from build123d import *

# Parameters (mm, degrees)
SKETCH1_W             = 6.35
SKETCH1_H             = 25.4
BOSS_EXTRUDE1_DEPTH   = 6.604
BOSS_EXTRUDE1_2_DEPTH = 6.604
SKETCH2_W             = 38.608
SKETCH2_H             = 25.4
BOSS_EXTRUDE2_DEPTH   = 5.08
SKETCH3_W             = 13.97
SKETCH3_H             = 6.35
BOSS_EXTRUDE3_DEPTH   = 6.604
SKETCH4_R             = 2.159
CUT_EXTRUDE1_DEPTH    = 2.54
SKETCH5_R             = 1.7018
BOSS_EXTRUDE4_DEPTH   = 11.684
FILLET1_R             = 6.35
FILLET2_R             = 3.81
FILLET3_R             = 1.27


with BuildPart() as part:
    # Sketch1 → Boss-Extrude1 (new body)
    with BuildSketch(Plane(origin=(0, 0, 0), x_dir=(1, 0, 0), z_dir=(0, 1, 0))):
        with Locations((16.129, 12.7)):
            Rectangle(SKETCH1_W, SKETCH1_H)
    extrude(amount=BOSS_EXTRUDE1_DEPTH)



with BuildPart() as body_2:
    # Sketch1 → Boss-Extrude1 2 (new body)
    with BuildSketch(Plane(origin=(0, 0, 0), x_dir=(1, 0, 0), z_dir=(0, 1, 0))):
        with Locations((-16.129, 12.7)):
            Rectangle(SKETCH1_W, SKETCH1_H)
    extrude(amount=BOSS_EXTRUDE1_2_DEPTH)


with BuildPart() as part_1:
    add(part.part)

    add(body_2.part)  # Boss-Extrude2 merges body 2
    # Sketch2 → Boss-Extrude2 (add)
    with BuildSketch(Plane(origin=(0, 6.604, 0), x_dir=(1, 0, 0), z_dir=(0, 1, 0))):
        with Locations((0, 12.7)):
            Rectangle(SKETCH2_W, SKETCH2_H)
    extrude(amount=BOSS_EXTRUDE2_DEPTH)

    # Sketch3 → Boss-Extrude3 (add)
    with BuildSketch(Plane.XZ.offset(-6.604)):
        with Locations((0, -22.225)):
            Rectangle(SKETCH3_W, SKETCH3_H)
    extrude(amount=BOSS_EXTRUDE3_DEPTH)

    # Sketch4 → Cut-Extrude1 (cut)
    with BuildSketch(Plane.XY.offset(-19.05)):
        with Locations((3.81, 3.302)):
            Circle(SKETCH4_R)
        with Locations((-3.81, 3.302)):
            Circle(SKETCH4_R)
    extrude(amount=-CUT_EXTRUDE1_DEPTH, mode=Mode.SUBTRACT)

    # Sketch5 → Boss-Extrude4 (add)
    # profile 1 of 2: a face of its own
    with BuildSketch(Plane(origin=(0, 11.684, 0), x_dir=(1, 0, 0), z_dir=(0, 1, 0))):
        with BuildLine():
            Line((-19.304, 17.985297981), (-19.304, 7.414702019))
            ThreePointArc((-19.304, 7.414702019), (-30.335321913, 12.7), (-19.304, 17.985297981))
        make_face()
        with Locations(Location((-23.553521913, 12.7, 0), (0, 0, 270))):
            Circle(SKETCH5_R, mode=Mode.SUBTRACT)
    # profile 2 of 2: a face of its own
    with BuildSketch(Plane(origin=(0, 11.684, 0), x_dir=(1, 0, 0), z_dir=(0, 1, 0))):
        with BuildLine():
            Line((19.304, 17.985297981), (19.304, 7.414702019))
            ThreePointArc((19.304, 7.414702019), (30.335321913, 12.7), (19.304, 17.985297981))
        make_face()
        with Locations(Location((23.553521913, 12.7, 0), (0, 0, 270))):
            Circle(SKETCH5_R, mode=Mode.SUBTRACT)
    extrude(amount=-BOSS_EXTRUDE4_DEPTH)

    # Fillet1
    # the kernel refuses this fillet: 6.35 mm, written as the material it adds along each edge
    with BuildSketch(Plane(origin=(-19.304, 11.684, -7.414702019), x_dir=(0, 0, 1), z_dir=(0, -1, 0)), Plane(origin=(19.304, 11.684, -17.985297981), x_dir=(0, 0, -1), z_dir=(0, -1, 0))) as fillet1_piece_1:
        with BuildLine():
            CenterArc((7.678309884, 6.344526057), FILLET1_R, 189.180006139, 78.44078763)
            Line((1.409640703, 5.331467961), (1.28426732, 5.311206799))
            ThreePointArc((1.28426732, 5.311206799), (1.148418354, 2.548446621), (-0.098975618, 0.079579062))
            Line((-0.098975618, 0.079579062), (0, -0.127))
            ThreePointArc((0, -0.127), (3.707351009, -0.127), (7.409429861, -0.126890521))
            Line((7.409429861, -0.126890521), (7.414702019, 0))
        make_face()
    extrude(amount=11.684)
    with BuildSketch(Plane(origin=(-19.304, 11.684, -17.985297981), x_dir=(0, 0, -1), z_dir=(0, -1, 0)), Plane(origin=(19.304, 11.684, -7.414702019), x_dir=(0, 0, 1), z_dir=(0, -1, 0))) as fillet1_piece_2:
        with BuildLine():
            CenterArc((7.678309884, -6.344526057), FILLET1_R, 92.379206231, 78.44078763)
            Line((1.409640703, -5.331467961), (1.28426732, -5.311206799))
            ThreePointArc((1.28426732, -5.311206799), (1.148418354, -2.548446621), (-0.098975618, -0.079579062))
            Line((-0.098975618, -0.079579062), (0, 0.127))
            ThreePointArc((0, 0.127), (3.707351009, 0.127), (7.409429861, 0.126890521))
            Line((7.409429861, 0.126890521), (7.414702019, 0))
        make_face()
    extrude(amount=11.684)

    # Fillet2
    fillet2_edges = [part_1.edges().sort_by_distance(p)[0] for p in [
        (20.899978754, 11.684, -21.447709562),
        (-19.304, 5.842, 0),
        (0, 11.684, 0),
        (0, 11.684, -25.4),
        (19.304, 5.842, 0),
        (19.304, 5.842, -25.4),
        (-30.335321913, 11.684, -12.7),
        (30.335321913, 11.684, -12.7),
        (-20.899978754, 11.684, -3.952290438),
        (-20.899978754, 11.684, -21.447709562),
        (20.899978754, 11.684, -3.952290438),
    ]]
    fillet(fillet2_edges, radius=FILLET2_R)

    # Fillet3
    fillet3_edges = [part_1.edges().sort_by_distance(p)[0] for p in [
        (0, 6.604, -19.05),
    ]]
    fillet(fillet3_edges, radius=FILLET3_R)


solid = part_1.part
For this review, take the finished solid that the model builds, in its own axes (mm). A direction names the side the tool comes from. Give positions to 0.01 mm unless a question says otherwise; leave off trailing zeros. Loops run counter-clockwise (first coordinate to the right, second up) from the corner with the lowest first, then second, coordinate; pieces in that order, holes last.
Item 1: Tool access review of faces 1 (the cylindrical face through (5.78, 6.24, -18.67)), 2 (the cylindrical face through (-5.967, 3.397, -20.302)), 3 (the flat face through (-12.954, 3, -13)), 4 (the cylindrical face through (-1.23, 10.54, -24.31)): name each direction out of +Z, -Z, +X, -X, +Y, -Y from which nothing blocks a thin tool from reaching the whole face with its end or side.
Item 2: For line 1 along X through (y, z) = (5.5, -12.7); line 2 along X through (y, z) = (7, -12.7); line 3 along X through (y, z) = (1.75, -22) (3 decimals), list the stretches that pass through material, from the lowest coordinate up.
Item 3: Insertion check: pin 1 (3.5 mm diameter, centred on y = 3.5, z = -23, fed in from -X); pin 2 (1.3 mm diameter, centred on x = -4.5, y = 3, fed in from +Z); pin 3 (1.5 mm diameter, centred on x = -15.5, z = -18, fed in from -Y); pin 4 (1.5 mm diameter, centred on x = 22, z = -3, fed in from -Y). Each pin has a flat end and moves straight along its axis. Give the tip position at first contact, or say it passes through.
Item 4: Take a section at B-B, the plane x = 9.5. State the section outline as (y, z) points.
Item 5: Take a section at A-A, the plane y = 4.25. Give the number of separate pieces and of enclosed holes in the cut face, and give its area (3 significant figures).
Item 6: Draft analysis for pull direction Y (two halves, no side actions). For faces 5 (the flat face through (-20, 0, -13)), 6 (the cylindrical face through (22.044, 5.924, -11.915)), 7 (the flat face through (4, 3, -21.59)), 8 (the flat face through (-4, 3, -21.59)), state which applies: +Y half, -Y half, draft (parallel to the pull), parting line (faces both ways), or undercut.
Calculated:
1. face 1: +Z, -Y
1. face 2: +Z
1. face 3: +Z, -Z, -Y
1. face 4: -Z, +X, -X, +Y
2. line 1: x = -30.34 to -25.26, -21.85 to -12.95, 12.95 to 21.85, 25.26 to 30.34
2. line 2: x = -30.34 to -25.26, -21.85 to 21.85, 25.26 to 30.34
2. line 3: x = -20.462 to -12.954, -6.985 to 6.985, 12.954 to 20.462
3. pin 1: stops at x = -21.08
3. pin 2: stops at z = -21.59
3. pin 3: stops at y = 0
3. pin 4: passes through
4. outline: (6.6, -25.4) - (7.87, -25.4) arc R3.81 ccw to (11.68, -21.59) - (11.68, -3.81) arc R3.81 ccw to (7.87, 0) - (6.6, 0) - close
5. separate pieces: 3
5. enclosed holes: 2
5. area: 660 mm2
6. face 5: -Y half
6. face 6: draft
6. face 7: undercut
6. face 8: undercut
